Could you check a few things on this model? Use its own coordinates, in mm. A direction names the side the tool comes from. Give positions to 0.01 mm unless a question says otherwise; leave off trailing zeros. Order: outer loops, then holes, each group sorted by start corner. A loop starts at its lowest first (then second) coordinate and runs counter-clockwise, first axis right, second up. Notation, with made-up numbers: (36.25, -8) -> (57.25, -8) arc R27 cw to (57.25, 12) -> close; hole circle Ø1 at (-4, 72). An arc over 180 degrees is marked (long way). One line per item, written item: value.
```python
from build123d import *

# Parameters (mm, degrees)
BOSS_EXTRUDE1_DEPTH = 19.05


with BuildPart() as part:
    # Sketch1 → Boss-Extrude1 (new body)
    with BuildSketch(Plane.XY):
        with BuildLine():
            Line((157.234081882, 128.980548454), (154.716315658, 154.51789158))
            Line((154.716315658, 154.51789158), (164.195357535, 155.452445004))
            Line((164.195357535, 155.452445004), (166.6875, 130.175))
            add(Edge.make_bspline(
                [(0, 0), (73.666580622, 1.740675992), (181.188092361, 36.200835609), (166.6875, 130.175)],
                knots=[0, 0, 0, 0, 1, 1, 1, 1], degree=3))
            add(Edge.make_bspline(
                [(0, 0), (-73.666580622, 1.740675992), (-181.188092361, 36.200835609), (-166.6875, 130.175)],
                knots=[0, 0, 0, 0, 1, 1, 1, 1], degree=3))
            Line((-166.6875, 130.175), (-109.368223301, 711.556235093))
            Line((-109.368223301, 711.556235093), (-99.889181424, 710.621681669))
            Line((-99.889181424, 710.621681669), (-157.234081882, 128.980548454))
            add(Edge.make_bspline(
                [(0, 9.52776174), (-1.117611602, 9.555193192), (-3.340472897, 9.624755056), (-7.880039481, 9.827207732), (-13.652210416, 10.198958437), (-20.725459036, 10.840441372), (-30.303235723, 11.962316267), (-42.47749757, 13.875858033), (-57.165232888, 17.02314898), (-71.689613059, 21.050850851), (-90.515854195, 27.626537064), (-112.436111514, 38.157452487), (-130.643933928, 51.803557723), (-142.189146149, 64.564536934), (-149.192253507, 75.075537554), (-153.541361304, 84.674022673), (-156.058613173, 92.923629982), (-157.442658539, 99.418206789), (-158.29640922, 106.242287005), (-158.540175044, 112.221426054), (-158.437150466, 117.190167219), (-158.20642164, 121.010360535), (-157.881730698, 124.277278241), (-157.584058118, 126.601085874), (-157.415798733, 127.781927866), (-157.316566229, 128.446705395), (-157.261207353, 128.804756083), (-157.234081882, 128.980548454)],
                knots=[0.001057036, 0.001057036, 0.001057036, 0.001057036, 0.016679825, 0.032302613, 0.063548191, 0.094793768, 0.126039346, 0.1885305, 0.251021655, 0.31351281, 0.376003965, 0.500986274, 0.625968584, 0.688459739, 0.750950893, 0.813442048, 0.844687626, 0.875933203, 0.90717878, 0.938424358, 0.954047147, 0.969669935, 0.985292724, 0.993104118, 0.997009815, 0.998962664, 1.000915513, 1.000915513, 1.000915513, 1.000915513], degree=3))
            add(Edge.make_bspline(
                [(157.234081882, 128.980548454), (157.261207353, 128.804756083), (157.316566229, 128.446705395), (157.415798733, 127.781927866), (157.584058118, 126.601085874), (157.881730698, 124.277278241), (158.20642164, 121.010360535), (158.437150466, 117.190167219), (158.540175044, 112.221426054), (158.29640922, 106.242287005), (157.442658539, 99.418206789), (156.058613173, 92.923629982), (153.541361304, 84.674022673), (149.192253507, 75.075537554), (142.189146149, 64.564536934), (130.643933928, 51.803557723), (112.436111514, 38.157452487), (90.515854195, 27.626537064), (71.689613059, 21.050850851), (57.165232888, 17.02314898), (42.47749757, 13.875858033), (30.303235723, 11.962316267), (20.725459036, 10.840441372), (13.652210416, 10.198958437), (7.880039481, 9.827207732), (3.340472897, 9.624755056), (1.117611602, 9.555193192), (0, 9.52776174)],
                knots=[0.001057036, 0.001057036, 0.001057036, 0.001057036, 0.003009885, 0.004962733, 0.00886843, 0.016679825, 0.032302613, 0.047925402, 0.063548191, 0.094793768, 0.126039346, 0.157284923, 0.1885305, 0.251021655, 0.31351281, 0.376003965, 0.500986274, 0.625968584, 0.688459739, 0.750950893, 0.813442048, 0.875933203, 0.90717878, 0.938424358, 0.969669935, 0.985292724, 1.000915513, 1.000915513, 1.000915513, 1.000915513], degree=3))
        make_face()
    extrude(amount=BOSS_EXTRUDE1_DEPTH)


solid = part.part
```
1) For faces 4 (the flat face through (155.993, 141.57, 9.392)), 5 (the flat face through (-138.43, 416.8, 9.39)), which set-ups out of +Z, -Z, +X, -X, +Y, -Y let a thin tool reach every point of the face, with its end or its side?
Answer below:
face 4: +Z, -Z
face 5: +Z, -Z, -X, +Y
2) We'd pull the mould along Y, two halves only. Please class faces 1 (the flat face through (-128.16, 423.87, 9.39)), 2 (the flat face through (165.424, 142.991, 9.392)), 3 (the flat face through (-147, 252, 19.05)): +Y half, -Y half, draft (parallel to the pull), parting line (faces both ways), or undercut.
Answer below:
face 1: undercut
face 2: +Y half
face 3: draft
3) For P1, Ø3, axis at y = 178.5, z = 5, coming from the +X side; P2, Ø2, axis at y = 286.5, z = 3.5, coming from the -X side; P3, Ø1.5, axis at y = 169.5, z = 16.5, coming from the -X side, each with a flat end and sliding along its axis, tell me the tip position at first contact or that it passes through.
Answer below:
P1: stops at x = -152.2
P2: stops at x = -151.37
P3: stops at x = -162.88
4) If I drill on line 1 along X through (y, z) = (52, 6); line 2 along X through (y, z) = (148.5, 8.5); line 3 along Y through (x, z) = (-2, 13.75), over which ranges is the centre line in solid material (lowest first)?
Answer below:
line 1: x = -143.54 to -129.87, 129.87 to 143.54
line 2: x = -164.88 to -155.31, 155.31 to 164.88
line 3: y = 0.06 to 9.58
5) Suppose I cut it at A-A, the plane y = 649. Write out the boundary of the cut face in (x, z), then the cut area to 3 significant figures.
Answer below:
outline: (-115.54, 0) -> (-105.96, 0) -> (-105.96, 19.05) -> (-115.54, 19.05) -> close
area: 182 mm2
